For this review, take the finished solid that the model builds, in its own axes (mm). Face numbers are marked on the shaded views. A direction names the side the tool comes from. Give positions to 0.01 mm unless a question says otherwise; leave off trailing zeros. Write each loop counter-clockwise with the first axis right and the second up, starting at its lowest first coordinate (ties: lowest second). Pieces come first, ordered by that corner, then holes. Notation, with made-up numbers: (50.25, -32) -> (106.25, -32) arc R27 cw to (106.25, 0) -> close; hole circle Ø5 at (-5.75, 58). An arc over 180 degrees is marked (long way). Answer as CSV lines item,"result".
```python
from build123d import *

# Parameters (mm, degrees)
F1_DEPTH = 25
F2_R     = 20
F3_DEPTH = 50.001
F4_R     = 15
F5_DEPTH = 50
F6_W     = 30
F6_H     = 45
F7_DEPTH = 26


# Not quite as in the source:
# - a pattern or mirror of a feature is missing from the dataset's text; its kind, count and spacing are read off the source's solid


with BuildPart() as f1:
    # F0 (on Right) → F1 (new body, symmetric)
    with BuildSketch(Plane.YZ):
        Polygon((-45, 0), (0, 0), (45, 0), (45, 10), (30, 40), (25, 40), (25, 70), (0, 70), (-25, 70), (-25, 40), (-30, 40), (-45, 10), align=None)
    extrude(amount=F1_DEPTH, both=True)

    # F2 (on face) → F3 (cut, through all)
    with BuildSketch(Plane.YZ.offset(25)):
        Circle(F2_R)
    extrude(amount=-F3_DEPTH, mode=Mode.SUBTRACT)

    # F4 (on face) → F5 (join)
    with BuildSketch(Plane.YZ.offset(25)):
        with Locations((0, 70)):
            Circle(F4_R)
    extrude(amount=-F5_DEPTH)

    # F6 (on face) → F7 (cut)
    with BuildSketch(Plane.XZ.offset(45)):
        with Locations((0, 47.5)):
            Rectangle(F6_W, F6_H)
    f7 = extrude(amount=-F7_DEPTH, mode=Mode.SUBTRACT)

    # F7_copies: F7 across plane
    add(f7.mirror(Plane.ZX), mode=Mode.SUBTRACT)


solid = f1.part
```
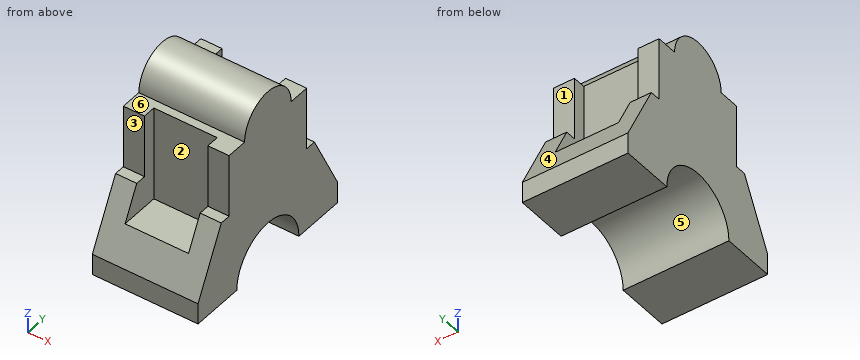
Q1. To check wall thickness, follow probe 1 along X at (y, z) = (20.5, 43); probe 2 along Y at (x, z) = (0, 37); probe 3 along Y at (x, z) = (-19.5, 48). State the ranges of each line that lie inside material, in increasing order. Write a range as [from, to].
Answer block:
probe 1,"x = [-25, -15], [15, 25]"
probe 2,"y = [-19, 19]"
probe 3,"y = [-25, 25]"
Q2. Draft analysis for pull direction Y (two halves, no side actions). For the marked faces 4, 5 and 6, state which applies: released by +Y, released by -Y, zero draft, split by the parting line, or undercut.
Answer block:
face 4,"released by +Y"
face 5,"undercut"
face 6,"zero draft"
Q3. For the marked faces 1, 2 and 3, list the 3-axis set-ups (+Z, -Z, +X, -X, +Y, -Y) from which the entire face can be reached by the end or side of a thin tool; tool diameter is ignored.
Answer block:
face 1,"+Z, +X, -X, +Y"
face 2,"+Z, -Y"
face 3,"+Z, +X, -X, -Y"
Q4. Add section A-A (x = -20.5). Write out the cut boundary in (y, z).
Answer block:
outline,"(-45, 0) -> (-20, 0) arc R20 cw to (20, 0) -> (45, 0) -> (45, 10) -> (30, 40) -> (25, 40) -> (25, 70) -> (15, 70) arc R15 ccw to (-15, 70) -> (-25, 70) -> (-25, 40) -> (-30, 40) -> (-45, 10) -> close"
Q5. Add section C-C (y = 0). Write out the cut boundary in (x, z), plus the area to 3 significant figures.
Answer block:
outline,"(-25, 20) -> (25, 20) -> (25, 85) -> (-25, 85) -> close"
area,"3,250 mm2"
Q6. Add section D-D (x = 12). Write out the cut boundary in (y, z).
Answer block:
outline,"(-45, 0) -> (-20, 0) arc R20 cw to (20, 0) -> (45, 0) -> (45, 10) -> (37.5, 25) -> (19, 25) -> (19, 70) -> (15, 70) arc R15 ccw to (-15, 70) -> (-19, 70) -> (-19, 25) -> (-37.5, 25) -> (-45, 10) -> close"
Q7. Clearance check with flat-ended pins moving along their axes: pin 1 (1.5 mm diameter, centred on x = 22, y = -27, fed in from +Z); pin 2 (15 mm diameter, centred on x = 4, z = 52.5, fed in from -Y); pin 3 (3 mm diameter, centred on x = 20, z = 55, fed in from +Y). State where each tip first meets the part, or that it passes through.
Answer block:
pin 1,"stops at z = 40"
pin 2,"stops at y = -19"
pin 3,"stops at y = 25"
Q8. Add section B-B (z = 57). Write out the cut boundary in (x, y).
Answer block:
outline,"(-25, -25) -> (-15, -25) -> (-15, -19) -> (15, -19) -> (15, -25) -> (25, -25) -> (25, 25) -> (15, 25) -> (15, 19) -> (-15, 19) -> (-15, 25) -> (-25, 25) -> close"
